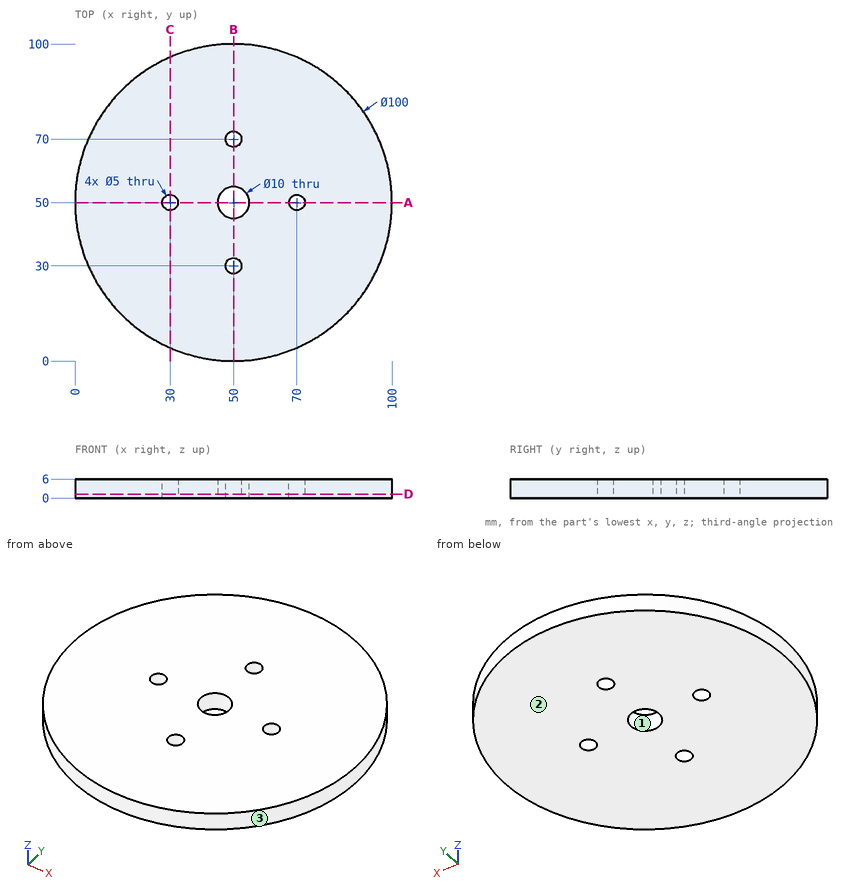
Check sheet for the drawn part. Datum: minimum x, y, z corner. Units: mm. Round coordinates to 2 decimals unless told otherwise and drop trailing zeros. Loops run counter-clockwise (first coordinate to the right, second up) from the corner with the lowest first, then second, coordinate; pieces in that order, holes last. Notation, with made-up numbers: (65.5, 6) -> (115.5, 6) arc R5 ccw to (115.5, 15) -> close; hole circle Ø7 at (0, 42). An arc over 180 degrees is marked (long way). Put each result on its own line as item: value. Start each with the question number.
1. Draft check along Y on the marked faces 1, 2 and 3. Enter one of: +Y half, -Y half, draft (parallel to the pull), parting line (faces both ways), or undercut.
2. Section check A-A (y = 50). Enter the section's corners in (x, z).
3. Gauge pin test, flat ends, axial feed: pin 1 (3 mm diameter, centred on x = 19.5, y = 72.5, fed in from -Z); pin 2 (3 mm diameter, centred on x = 23.5, z = 3.5, fed in from +Y). Record the tip position at first contact, or that the pin passes through.
4. Section check D-D (z = 1.25). Enter the section's corners in (x, y), plus the area to 3 significant figures.
5. Section check C-C (x = 30). Enter the section's corners in (y, z).
6. Scan lines: probe 1 along Y at (x, z) = (50, 5.25); probe 2 along Y at (x, z) = (69, 5.5); probe 3 along Y at (x, z) = (70, 3.1). Record each from-to range of solid material in increasing order.
Findings:
1. face 1: undercut
1. face 2: draft
1. face 3: parting line
2. outline: (0, 0) -> (27.5, 0) -> (27.5, 6) -> (0, 6) -> close; (32.5, 0) -> (45, 0) -> (45, 6) -> (32.5, 6) -> close; (55, 0) -> (67.5, 0) -> (67.5, 6) -> (55, 6) -> close; (72.5, 0) -> (100, 0) -> (100, 6) -> (72.5, 6) -> close
3. pin 1: stops at z = 0
3. pin 2: stops at y = 93.3
4. outline: circle Ø100 at (50, 50); hole circle Ø5 at (30, 50); hole circle Ø10 at (50, 50); hole circle Ø5 at (50, 30); hole circle Ø5 at (50, 70); hole circle Ø5 at (70, 50)
4. area: 7,700 mm^2
5. outline: (4.17, 0) -> (47.5, 0) -> (47.5, 6) -> (4.17, 6) -> close; (52.5, 0) -> (95.83, 0) -> (95.83, 6) -> (52.5, 6) -> close
6. probe 1: y = 0 to 27.5, 32.5 to 45, 55 to 67.5, 72.5 to 100
6. probe 2: y = 3.75 to 47.71, 52.29 to 96.25
6. probe 3: y = 4.17 to 47.5, 52.5 to 95.83
